CAD build for the part. Positions are in the model's coordinates, mm. Give positions to 0.01 mm unless a question says otherwise; leave off trailing zeros. Loops run counter-clockwise (first coordinate to the right, second up) from the corner with the lowest first, then second, coordinate; pieces in that order, holes last.
Autodesk Inventor part; units mm, degrees
ref_plane "YZ Plane" through (0, 0, 0) normal (1, 0, 0) x (0, 1, 0)
ref_plane "XZ Plane" through (0, 0, 0) normal (0, 1, 0) x (-1, 0, 0)
ref_plane "XY Plane" through (0, 0, 0) normal (0, 0, 1) x (1, 0, 0)
sketch "Эскиз1" plane through (0, 0, 0) normal (0, 0, 1) x (1, 0, 0)
  line L0 (15.9926, -16.8371) -> (138.9926, -16.8371)
  line L1 (139.9926, -17.8371) -> (139.9926, -45.3371)
  line L2 (139.9926, -45.3371) -> (138.4926, -45.3371)
  line L3 (138.4926, -45.3371) -> (138.4926, -57.3371)
  line L4 (138.4926, -57.3371) -> (139.9926, -57.3371)
  line L5 (139.9926, -57.3371) -> (139.9926, -84.8371)
  line L6 (138.9926, -85.8371) -> (15.9926, -85.8371)
  line L7 (14.9926, -84.8371) -> (14.9926, -57.3371)
  line L8 (14.9926, -57.3371) -> (16.4926, -57.3371)
  line L9 (16.4926, -57.3371) -> (16.4926, -45.3371)
  line L10 (16.4926, -45.3371) -> (14.9926, -45.3371)
  line L11 (14.9926, -45.3371) -> (14.9926, -17.8371)
  circle A0 centre (25.4926, -51.3371) radius 6
  circle A1 centre (129.4926, -51.3371) radius 6
  line L12 (33.4926, -57.3371) -> (33.4926, -45.3371)
  line L13 (33.4926, -45.3371) -> (37.4926, -45.3371)
  line L14 (37.4926, -45.3371) -> (37.4926, -57.3371)
  line L15 (37.4926, -57.3371) -> (33.4926, -57.3371)
  arc A2 (44.4926, -48.8371) -> (40.4926, -48.8371) centre (42.4926, -48.8371) ccw
  arc A3 (40.4926, -53.8371) -> (44.4926, -53.8371) centre (42.4926, -53.8371) ccw
  line L16 (44.4926, -53.8371) -> (44.4926, -48.8371)
  line L17 (40.4926, -53.8371) -> (40.4926, -48.8371)
  circle A4 centre (77.4926, -51.3371) radius 10
  line L18 (102.4926, -43.3371) -> (102.4926, -40.3371)
  line L19 (102.4926, -40.3371) -> (90.4926, -40.3371)
  line L20 (90.4926, -40.3371) -> (90.4926, -43.3371)
  line L21 (90.4926, -43.3371) -> (102.4926, -43.3371)
  circle A5 centre (77.4926, -20.8371) radius 2
  circle A6 centre (65.4926, -20.8371) radius 2
  circle A7 centre (89.4926, -20.8371) radius 2
  circle A8 centre (82.4926, -26.3371) radius 2
  circle A9 centre (118.4926, -20.8371) radius 2
  line L22 (106.4926, -61.8371) -> (106.4926, -68.3371)
  line L23 (106.4926, -68.3371) -> (102.4926, -68.3371)
  line L24 (102.4926, -68.3371) -> (102.4926, -76.3371)
  line L25 (102.4926, -76.3371) -> (106.4926, -76.3371)
  line L26 (115.4926, -61.8371) -> (106.4926, -61.8371)
  line L27 (115.4926, -68.3371) -> (115.4926, -61.8371)
  line L28 (106.4926, -76.3371) -> (106.4926, -82.8371)
  line L29 (106.4926, -82.8371) -> (115.4926, -82.8371)
  line L30 (115.4926, -82.8371) -> (115.4926, -76.3371)
  line L31 (115.4926, -76.3371) -> (119.4926, -76.3371)
  line L32 (119.4926, -68.3371) -> (115.4926, -68.3371)
  line L33 (119.4926, -76.3371) -> (119.4926, -68.3371)
  arc A10 (15.9926, -16.8371) -> (14.9926, -17.8371) centre (15.9926, -17.8371) ccw
  arc A11 (14.9926, -84.8371) -> (15.9926, -85.8371) centre (15.9926, -84.8371) ccw
  arc A12 (138.9926, -85.8371) -> (139.9926, -84.8371) centre (138.9926, -84.8371) ccw
  arc A13 (139.9926, -17.8371) -> (138.9926, -16.8371) centre (138.9926, -17.8371) ccw
  circle A14 centre (96.4926, -26.3371) radius 2
  circle A15 centre (58.4926, -26.3371) radius 2
  circle A16 centre (72.4926, -26.3371) radius 2
  circle A17 centre (36.4926, -20.8371) radius 2
  line L34 (102.4926, -59.3371) -> (102.4926, -62.3371)
  line L35 (102.4926, -62.3371) -> (90.4926, -62.3371)
  line L36 (90.4926, -62.3371) -> (90.4926, -59.3371)
  line L37 (90.4926, -59.3371) -> (102.4926, -59.3371)
  line L38 (52.4926, -43.3371) -> (52.4926, -40.3371)
  line L39 (52.4926, -40.3371) -> (64.4926, -40.3371)
  line L40 (64.4926, -40.3371) -> (64.4926, -43.3371)
  line L41 (64.4926, -43.3371) -> (52.4926, -43.3371)
  line L42 (52.4926, -59.3371) -> (52.4926, -62.3371)
  line L43 (64.4926, -59.3371) -> (52.4926, -59.3371)
  line L44 (64.4926, -62.3371) -> (64.4926, -59.3371)
  line L45 (52.4926, -62.3371) -> (64.4926, -62.3371)
  line L46 (121.4926, -57.3371) -> (121.4926, -45.3371)
  line L47 (121.4926, -45.3371) -> (117.4926, -45.3371)
  line L48 (117.4926, -45.3371) -> (117.4926, -57.3371)
  line L49 (117.4926, -57.3371) -> (121.4926, -57.3371)
  arc A18 (114.4926, -48.8371) -> (110.4926, -48.8371) centre (112.4926, -48.8371) ccw
  arc A19 (110.4926, -53.8371) -> (114.4926, -53.8371) centre (112.4926, -53.8371) ccw
  line L50 (110.4926, -53.8371) -> (110.4926, -48.8371)
  line L51 (114.4926, -53.8371) -> (114.4926, -48.8371)
  line L52 (82.4926, -26.3371) -> (82.4926, -26.3371)
  circle A20 centre (77.4926, -81.8371) radius 2
  circle A21 centre (65.4926, -81.8371) radius 2
  circle A22 centre (89.4926, -81.8371) radius 2
  circle A23 centre (82.4926, -76.3371) radius 2
  circle A24 centre (118.4926, -81.8371) radius 2
  circle A25 centre (96.4926, -76.3371) radius 2
  circle A26 centre (58.4926, -76.3371) radius 2
  circle A27 centre (72.4926, -76.3371) radius 2
  circle A28 centre (36.4926, -81.8371) radius 2
  line L53 (39.4926, -61.8371) -> (48.4926, -61.8371)
  line L54 (39.4926, -68.3371) -> (39.4926, -61.8371)
  line L55 (48.4926, -61.8371) -> (48.4926, -68.3371)
  line L56 (48.4926, -68.3371) -> (52.4926, -68.3371)
  line L57 (52.4926, -68.3371) -> (52.4926, -76.3371)
  line L58 (52.4926, -76.3371) -> (48.4926, -76.3371)
  line L59 (48.4926, -82.8371) -> (39.4926, -82.8371)
  line L60 (48.4926, -76.3371) -> (48.4926, -82.8371)
  line L61 (39.4926, -82.8371) -> (39.4926, -76.3371)
  line L62 (39.4926, -76.3371) -> (35.4926, -76.3371)
  line L63 (35.4926, -68.3371) -> (39.4926, -68.3371)
  line L64 (35.4926, -76.3371) -> (35.4926, -68.3371)
  point P0 (0, 0)
  point P1 (14.9926, -16.8371)
  point P2 (139.9926, -16.8371)
  point P3 (139.9926, -85.8371)
  point P4 (34.4926, -62.3371)
  point P5 (51.4926, -81.3371)
  point P6 (119.9926, -62.3371)
  point P7 (102.9926, -81.3371)
  point P8 (118.4926, -81.3371)
extrude "Выдавливание3" add sketch "Эскиз1" along normal blind 2
properties part number "Зад"
1. Pull direction Y, two halves, no side cores. Call faces 1 (the face through (57.02, -27.69, 0.99)), 2 (the face through (38.4, -21.44, 0.99)), 3 (the face through (63, -51, 2)): released by +Y, released by -Y, zero draft, split by the parting line, or undercut.
Responses:
face 1: undercut
face 2: undercut
face 3: zero draft
2. Probe line 1 along X through (y, z) = (-64, 1.7); line 2 along X through (y, z) = (-74, 1.55); line 3 along Y through (x, z) = (55.5, 1.6). List the from-to ranges inside material, lowest first.
Responses:
line 1: x = 14.99 to 39.49, 48.49 to 106.49, 115.49 to 139.99
line 2: x = 14.99 to 35.49, 52.49 to 102.49, 119.49 to 139.99
line 3: y = -85.84 to -62.34, -59.34 to -43.34, -40.34 to -16.84
3. Saw through at C-C, the plane x = 82.5. List the corners of the cut face in (y, z), and give its area (3 significant figures).
Responses:
outline: (-85.84, 0) - (-78.34, 0) - (-78.34, 2) - (-85.84, 2) - close; (-74.34, 0) - (-59.99, 0) - (-59.99, 2) - (-74.34, 2) - close; (-42.68, 0) - (-28.34, 0) - (-28.34, 2) - (-42.68, 2) - close; (-24.34, 0) - (-16.84, 0) - (-16.84, 2) - (-24.34, 2) - close
area: 87.4 mm2
4. Saw through at B-B, the plane x = 54. List the corners of the cut face in (y, z).
Responses:
outline: (-85.84, 0) - (-62.34, 0) - (-62.34, 2) - (-85.84, 2) - close; (-59.34, 0) - (-43.34, 0) - (-43.34, 2) - (-59.34, 2) - close; (-40.34, 0) - (-16.84, 0) - (-16.84, 2) - (-40.34, 2) - close
5. Saw through at A-A, the plane y = -65. List the corners of the cut face in (x, z).
Responses:
outline: (14.99, 0) - (39.49, 0) - (39.49, 2) - (14.99, 2) - close; (48.49, 0) - (106.49, 0) - (106.49, 2) - (48.49, 2) - close; (115.49, 0) - (139.99, 0) - (139.99, 2) - (115.49, 2) - close
6. Drop flat-ended pins along their axis: pin 1 (4 mm diameter, centred on x = 84, y = -39, fed in from -Z); pin 2 (0.6 mm diameter, centred on y = -50.5, z = 1, fed in from -X); pin 3 (1 mm diameter, centred on y = -51, z = 0.5, fed in from +X). Give the stop position or say it passes through.
Responses:
pin 1: stops at z = 0
pin 2: stops at x = 16.49
pin 3: stops at x = 138.49
7. Saw through at D-D, the plane x = 24.5. List the corners of the cut face in (y, z).
Responses:
outline: (-85.84, 0) - (-57.25, 0) - (-57.25, 2) - (-85.84, 2) - close; (-45.42, 0) - (-16.84, 0) - (-16.84, 2) - (-45.42, 2) - close
